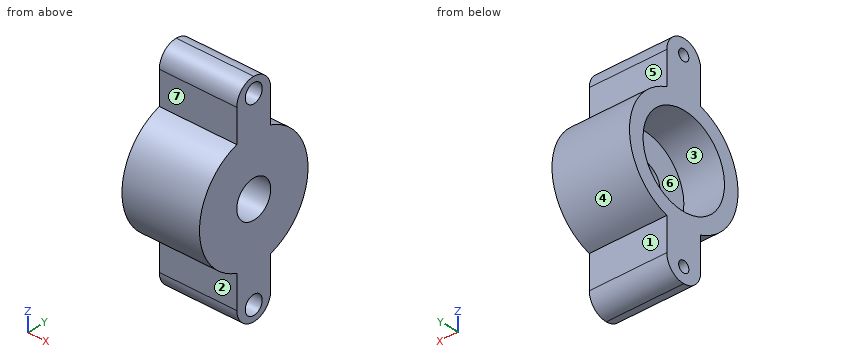
```python
from build123d import *

# Parameters (mm, degrees)
SKETCH1_W                = 70
SKETCH1_H                = 10
BOSS_EXTRUDE1_DEPTH      = 5
BOSS_EXTRUDE2_DEPTH      = 16
BOSS_EXTRUDE2_DEPTH_BACK = 5
SKETCH2_R                = 16
SKETCH3_W                = 70
SKETCH3_H                = 10
BOSS_EXTRUDE3_DEPTH      = 16
SKETCH4_R                = 2.5
CUT_EXTRUDE1_DEPTH       = 11
SKETCH5_R                = 1.5
CUT_EXTRUDE2_DEPTH       = 38
SKETCH6_R                = 12
CUT_EXTRUDE3_DEPTH       = 11
SKETCH7_R                = 5
CUT_EXTRUDE4_DEPTH       = 40
SKETCH8_W                = 6
SKETCH8_H                = 10
CUT_EXTRUDE5_DEPTH       = 40
FILLET1_R                = 5
FILLET2_R                = 5
FILLET3_R                = 5
FILLET4_R                = 5


with BuildPart() as part:
    # Sketch1 → Boss-Extrude1 (new body)
    with BuildSketch(Plane(origin=(0, 0, 0), x_dir=(0, 0, -1), z_dir=(1, 0, 0))):
        with Locations((35, 5)):
            Rectangle(SKETCH1_W, SKETCH1_H)
    extrude(amount=BOSS_EXTRUDE1_DEPTH)

    # Sketch2 → Boss-Extrude2 (add, two sides: drawn at the far end of the back side and taken through both)
    with BuildSketch(Plane(origin=(5, 0, 0), x_dir=(0, 0, -1), z_dir=(1, 0, 0)).offset(-BOSS_EXTRUDE2_DEPTH_BACK)):
        with Locations(Location((35, 5, 0), (0, 0, 161.790043136))):
            Circle(SKETCH2_R)
    extrude(amount=BOSS_EXTRUDE2_DEPTH + BOSS_EXTRUDE2_DEPTH_BACK)

    # Sketch3 → Boss-Extrude3 (add)
    with BuildSketch(Plane(origin=(5, 0, 0), x_dir=(0, 0, -1), z_dir=(1, 0, 0))):
        with Locations((35, 5)):
            Rectangle(SKETCH3_W, SKETCH3_H)
    extrude(amount=BOSS_EXTRUDE3_DEPTH)

    # Sketch4 → Cut-Extrude1 (cut)
    with BuildSketch(Plane(origin=(21, 0, 0), x_dir=(0, 0, -1), z_dir=(1, 0, 0))):
        with Locations((10, 5)):
            Circle(SKETCH4_R)
        with Locations((60, 5)):
            Circle(SKETCH4_R)
    extrude(amount=-CUT_EXTRUDE1_DEPTH, mode=Mode.SUBTRACT)

    # Sketch5 → Cut-Extrude2 (cut)
    with BuildSketch(Plane(origin=(21, 0, 0), x_dir=(0, 0, -1), z_dir=(1, 0, 0))):
        with Locations((10, 5)):
            Circle(SKETCH5_R)
        with Locations((60, 5)):
            Circle(SKETCH5_R)
    extrude(amount=-CUT_EXTRUDE2_DEPTH, mode=Mode.SUBTRACT)

    # Sketch6 → Cut-Extrude3 (cut)
    with BuildSketch(Plane.ZY):
        with Locations((-35, 5)):
            Circle(SKETCH6_R)
    extrude(amount=-CUT_EXTRUDE3_DEPTH, mode=Mode.SUBTRACT)

    # Sketch7 → Cut-Extrude4 (cut)
    with BuildSketch(Plane(origin=(21, 0, 0), x_dir=(0, 0, -1), z_dir=(1, 0, 0))):
        with Locations((35, 5)):
            Circle(SKETCH7_R)
    extrude(amount=-CUT_EXTRUDE4_DEPTH, mode=Mode.SUBTRACT)

    # Sketch8 → Cut-Extrude5 (cut)
    with BuildSketch(Plane.ZY):
        with Locations((-67, 5)):
            Rectangle(SKETCH8_W, SKETCH8_H)
        with Locations((-3, 5)):
            Rectangle(SKETCH8_W, SKETCH8_H)
    extrude(amount=-CUT_EXTRUDE5_DEPTH, mode=Mode.SUBTRACT)

    # Fillet1
    fillet1_edges = [part.edges().sort_by_distance(p)[0] for p in [
        (10.5, 10, -64),
    ]]
    fillet(fillet1_edges, radius=FILLET1_R)

    # Fillet2
    fillet2_edges = [part.edges().sort_by_distance(p)[0] for p in [
        (10.5, 10, -6),
    ]]
    fillet(fillet2_edges, radius=FILLET2_R)

    # Fillet3
    fillet3_edges = [part.edges().sort_by_distance(p)[0] for p in [
        (10.5, 0, -6),
    ]]
    fillet(fillet3_edges, radius=FILLET3_R - 0.0001)  # a hair under: the kernel refuses the full size

    # Fillet4
    fillet4_edges = [part.edges().sort_by_distance(p)[0] for p in [
        (10.5, 0, -64),
    ]]
    fillet(fillet4_edges, radius=FILLET4_R - 0.0001)  # a hair under: the kernel refuses the full size


solid = part.part
```
For this review, take the finished solid that the model builds, in its own axes (mm). Face numbers are marked on the shaded views. A direction names the side the tool comes from. Coordinates: 2 decimals unless noted, no trailing zeros. Write each loop counter-clockwise with the first axis right and the second up, starting at its lowest first coordinate (ties: lowest second). Pieces come first, ordered by that corner, then holes. Notation, with made-up numbers: (74, 20.5) - (117, 20.5) arc R4 ccw to (117, 24.5) - close; hole circle Ø1 at (8, 51). An arc over 180 degrees is marked (long way). Put each result on its own line as item: value.
1. Add section C-C, the plane y = -1. Give the boundary of the cut face in (x, z).
Values found:
outline: (0, -49.83) - (21, -49.83) - (21, -20.17) - (0, -20.17) - (0, -24.61) - (11, -24.61) - (11, -45.39) - (0, -45.39) - close
2. Add section D-D, the plane z = -28. Give the boundary of the cut face in (x, y), then the cut area to 3 significant figures.
Values found:
outline: (0, -9.39) - (21, -9.39) - (21, 19.39) - (0, 19.39) - (0, 14.75) - (11, 14.75) - (11, -4.75) - (0, -4.75) - close
area: 390 mm²
3. Add section A-A, the plane z = -35. Give the boundary of the cut face in (x, y).
Values found:
outline: (0, -11) - (21, -11) - (21, 0) - (11, 0) - (11, -7) - (0, -7) - close; (0, 17) - (11, 17) - (11, 10) - (21, 10) - (21, 21) - (0, 21) - close
4. Mouldability with a two-part tool opening along Y and no side actions: class the marked faces 5, 6 and 7 as released by +Y, released by -Y, zero draft, split by the parting line, or undercut.
Values found:
face 5: released by +Y
face 6: undercut
face 7: released by -Y
5. Wall thickness on probe 1 along Y at (x, z) = (7.75, -10); probe 2 along Y at (x, z) = (14.5, -13); probe 3 along Y at (x, z) = (9.5, -44): over which ranges is each line inside the solid? List them lowest first.
Values found:
probe 1: 0.1 to 3.5, 6.5 to 9.9
probe 2: 0 to 10
probe 3: -8.23 to -2.94, 12.94 to 18.23
6. Machinability: for the marked faces 1, 2, 3 and 4, which of the approach directions +Z, -Z, +X, -X, +Y, -Y give a long, thin tool a straight path to every point of the face, cutting with its end or side? Answer none if there is none.
Values found:
face 1: -Z, +X, -X, +Y
face 2: -Z, +X, -X, -Y
face 3: -X
face 4: +X, -X, +Y
7. Add section B-B, the plane x = 12.5. Count the separate pieces of the cut face and the enclosed holes in it, then the cut area to 3 significant figures.
Values found:
separate pieces: 1
enclosed holes: 3
area: 930 mm²
8. For pin 1 (4 mm diameter, centred on x = 8.5, z = -42.5, fed in from +Y) (3 decimals); pin 2 (7 mm diameter, centred on x = 11.5, z = -15, fed in from +Y); pin 3 (7 mm diameter, centred on y = 1.5, z = -36, fed in from -X), all flat-tipped, find the tip position at first contact; note any pin that passes through.
Values found:
pin 1: y = 20.025
pin 2: y = 10
pin 3: x = 11
